Geometry: final body of the model. Coordinates: model frame, mm. A direction names the side the tool comes from. Coordinates: 2 decimals unless noted, no trailing zeros. Order: outer loops, then holes, each group sorted by start corner. A loop starts at its lowest first (then second) coordinate and runs counter-clockwise, first axis right, second up. Notation, with made-up numbers: (4, 54) - (45, 54) arc R24 ccw to (45, 75) - close; hole circle Ø1 at (64, -2). An arc over 180 degrees is marked (long way). Use a Markdown table: item, result. Add a question column.
```python
from build123d import *

# Parameters (mm, degrees)
CUT_EXTRUDE1_DEPTH      = 78.771299333
CUT_EXTRUDE1_DEPTH_BACK = 78.771299333


with BuildPart() as part:
    # Sketch1 → Revolve1 (revolve)
    with BuildSketch(Plane.XY, mode=Mode.PRIVATE) as revolve1_sk:
        Polygon((0, 0), (63.5, 0), (63.5, 25.4), (44.45, 31.75), (19.05, 31.75), (0, 25.4), align=None)
    revolve(revolve1_sk.sketch.rotate(Axis((0, 0, 0), (1, 0, 0)), 90), axis=Axis((0, 0, 0), (1, 0, 0)))

    # Sketch2 → Cut-Extrude1 (cut, two sides: drawn at the far end of the back side and taken through both)
    with BuildSketch(Plane.ZY.offset(-CUT_EXTRUDE1_DEPTH_BACK)):
        Polygon((-3.666174209, 6.35), (-7.332348419, 0), (-3.666174209, -6.35), (3.666174209, -6.35), (7.332348419, 0), (3.666174209, 6.35), align=None)
    extrude(amount=CUT_EXTRUDE1_DEPTH + CUT_EXTRUDE1_DEPTH_BACK, mode=Mode.SUBTRACT)


solid = part.part
```
1) Section C-C (x = 12). Return loops of the section in (y, z).
2) Pin query (flat end, axial travel): pin 1 (12 mm diameter, centred on y = 4, z = -7.5, fed in from -X); pin 2 (1 mm diameter, centred on x = 15.5, z = -19, fed in from -Y); pin 3 (2 mm diameter, centred on x = 41.5, z = -1, fed in from +Y); pin 4 (2 mm diameter, centred on x = 52, y = -21, fed in from +Z). Return the tip coordinate at first contact, or that it passes through.
3) Ray query, line 1 along Y through (x, z) = (42, 0.5); line 2 along Z through (x, y) = (42, -1) (3 decimals); line 3 along Y through (x, z) = (18, 3.5). Return the intervals inside material, ascending.
4) Set-up query: faces 1 (the face through (32.194, 3.219, -5.474)), 2 (the face through (0.925, 22.808, 11.863)). Return all of +Z, -Z, +X, -X, +Y, -Y with unobstructed straight access to the full face (end or side cutting, diameter ignored); none if empty.
5) Section A-A (z = 0). Return loops of the section in (x, y).
6) Section B-B (x = 42.5). Return loops of the section in (y, z).
7) Draft query along Y for faces 3 (the face through (32, 6.35, 0)), 4 (the face through (63.5, 5, -5)), 5 (the face through (31.572, 30.995, -6.883)). Return one class per face: pulls with the +Y half, pulls with the -Y half, needs draft (parallel to the pull), parting line crosses it, or undercut.
Values follow:
| question | item | result |
|---|---|---|
| 1 | outline | circle Ø58.8 at (0, 0); hole (-6.35, -3.67) - (0, -7.33) - (6.35, -3.67) - (6.35, 3.67) - (0, 7.33) - (-6.35, 3.67) - close |
| 2 | pin 1 | stops at x = 0 |
| 2 | pin 2 | stops at y = -24.39 |
| 2 | pin 3 | stops at y = 31.75 |
| 2 | pin 4 | stops at z = 21.43 |
| 3 | line 1 | y = -31.75 to -6.35, 6.35 to 31.75 |
| 3 | line 2 | z = -31.734 to -6.755, 6.755 to 31.734 |
| 3 | line 3 | y = -31.2 to -6.35, 6.35 to 31.2 |
| 4 | face 1 | +X, -X |
| 4 | face 2 | -X |
| 5 | outline | (0, -25.4) - (19.05, -31.75) - (44.45, -31.75) - (63.5, -25.4) - (63.5, -6.35) - (0, -6.35) - close; (0, 6.35) - (63.5, 6.35) - (63.5, 25.4) - (44.45, 31.75) - (19.05, 31.75) - (0, 25.4) - close |
| 6 | outline | circle Ø63.5 at (0, 0); hole (-6.35, -3.67) - (0, -7.33) - (6.35, -3.67) - (6.35, 3.67) - (0, 7.33) - (-6.35, 3.67) - close |
| 7 | face 3 | undercut |
| 7 | face 4 | needs draft |
| 7 | face 5 | parting line crosses it |
